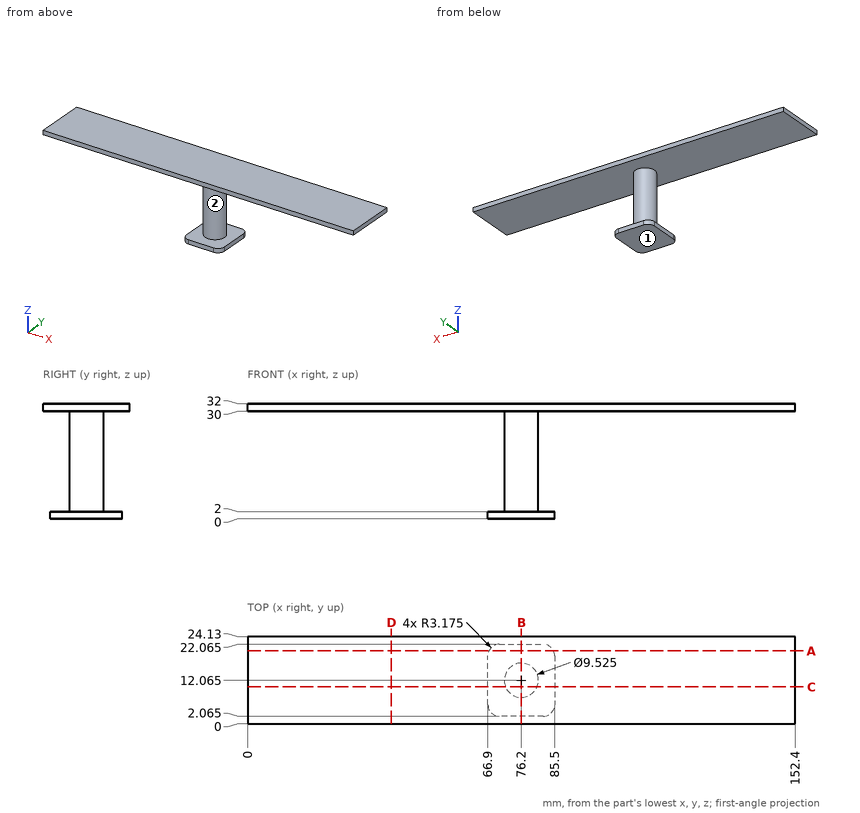
Geometry: see drawing. Coordinates: mm, zero at the bounding-box minimum. A direction names the side the tool comes from. Coordinates: 2 decimals unless noted, no trailing zeros. Order: outer loops, then holes, each group sorted by start corner. A loop starts at its lowest first (then second) coordinate and runs counter-clockwise, first axis right, second up. Notation, with made-up numbers: M 37.5,40 L 95.5,40 A31 ccw 95.5,68 Z; hole C 35,67.25 d5. An arc over 180 degrees is marked long. Write each question's results on one line, items separated by ' | '. Start each with the question number.
1) Access query for the marked faces 1 and 2. Directions: +Z, -Z, +X, -X, +Y, -Y. A direction counts if a zero-diameter tool reaches every point of the face in a straight line with its end or side. Return the directions, or none.
2) Section query D-D (x = 40). Return the cut outline in (y, z).
3) Section query A-A (y = 20.25). Return the cut outline in (x, z), plus the area to 3 significant figures.
4) Section query C-C (y = 10.25). Return the cut outline in (x, z), plus the area to 3 significant figures.
5) Section query B-B (x = 76.2). Return the cut outline in (y, z) (1 decimal), plus the area to 3 significant figures.
6) Line query: line 1 (Z direction, x = 77, y = 18.5); line 2 (Z direction, x = 99, y = 5.75); line 3 (X direction, y = 11, z = 1.5). Output: solid intervals per line, ascending. Write a range as from..to.
7) Contact query for flat-ended pins moving along their axis: pin 1 Ø1 at (x, y) = (132.5, 6) entering from -Z; pin 2 Ø2 at (y, z) = (10, 1) entering from +X; pin 3 Ø10 at (y, z) = (19, 8) entering from +X. Output: stop coordinate, or through.
Answers:
1) face 1: -Z, +X, -X, +Y, -Y | face 2: none
2) outline: M 0,30 L 24.13,30 L 24.13,32 L 0,32 Z
3) outline: M 0,30 L 152.4,30 L 152.4,32 L 0,32 Z; M 67.21,0 L 85.19,0 L 85.19,2 L 67.21,2 Z | area: 341 mm^2
4) outline: M 0,30 L 71.8,30 L 71.8,2 L 66.9,2 L 66.9,0 L 85.5,0 L 85.5,2 L 80.6,2 L 80.6,30 L 152.4,30 L 152.4,32 L 0,32 Z | area: 589 mm^2
5) outline: M 0,30 L 7.3,30 L 7.3,2 L 2.1,2 L 2.1,0 L 22.1,0 L 22.1,2 L 16.8,2 L 16.8,30 L 24.1,30 L 24.1,32 L 0,32 Z | area: 355 mm^2
6) line 1: z = 0..2, 30..32 | line 2: z = 30..32 | line 3: x = 66.9..85.5
7) pin 1: stops at z = 30 | pin 2: stops at x = 85.5 | pin 3: stops at x = 80.55
